The figure shows three views and two pictorial views of one solid part (mm, origin at its lowest corner). Answer the questions. A direction names the side the tool comes from. Coordinates: 2 decimals unless noted, no trailing zeros. Loops run counter-clockwise (first coordinate to the right, second up) from the corner with the lowest first, then second, coordinate; pieces in that order, holes last. Notation, with made-up numbers: M 12,-16 L 25,-16 A17 cw 25,5 Z; hole C 22.5,59 d5. An arc over 180 degrees is marked long. Return JSON: item names as keys, results as strings. Group by question number.
1. The mould has two halves that part along X. Classify the marked faces 4, 5 and 6: pulls with the +X half, pulls with the -X half, needs draft (parallel to the pull), parting line crosses it, or undercut.
2. Given P1, Ø4.5, axis at x = 39, z = 47, coming from the +Y side; P2, Ø1, axis at y = 31, z = 44.5, coming from the -X side; P3, Ø6, axis at y = 10.5, z = 32.5, coming from the -X side, each flat-ended and moving along its own axis, determine where each tip first touches the part or whether it passes through.
3. Section C-C (z = 11.5) is taken. Write down the section's boundary in (x, y), then the cut area to 3 significant figures.
4. Section B-B (y = 45) is taken. Write down the section's boundary in (x, z), then the cut area to 3 significant figures.
5. Section D-D (x = 66) is taken. Write down the section's boundary in (y, z) (1 decimal).
6. Section A-A (z = 28.5) is taken. Write down the section's boundary in (x, y), then the cut area to 3 significant figures.
7. Straight lines are drawn through the part: L1, parallel to Z at x = 66, y = 66.5; L2, parallel to Y at x = 49.5, z = 46.5; L3, parallel to Y at x = 24, z = 32.5. For each, find the intervals that lie inside material, in ascending order. Write a range as from..to.
8. Which of the six approach directions +Z, -Z, +X, -X, +Y, -Y give full straight-line access (tool end or side, diameter ignored) to the marked faces 1, 2 and 3?
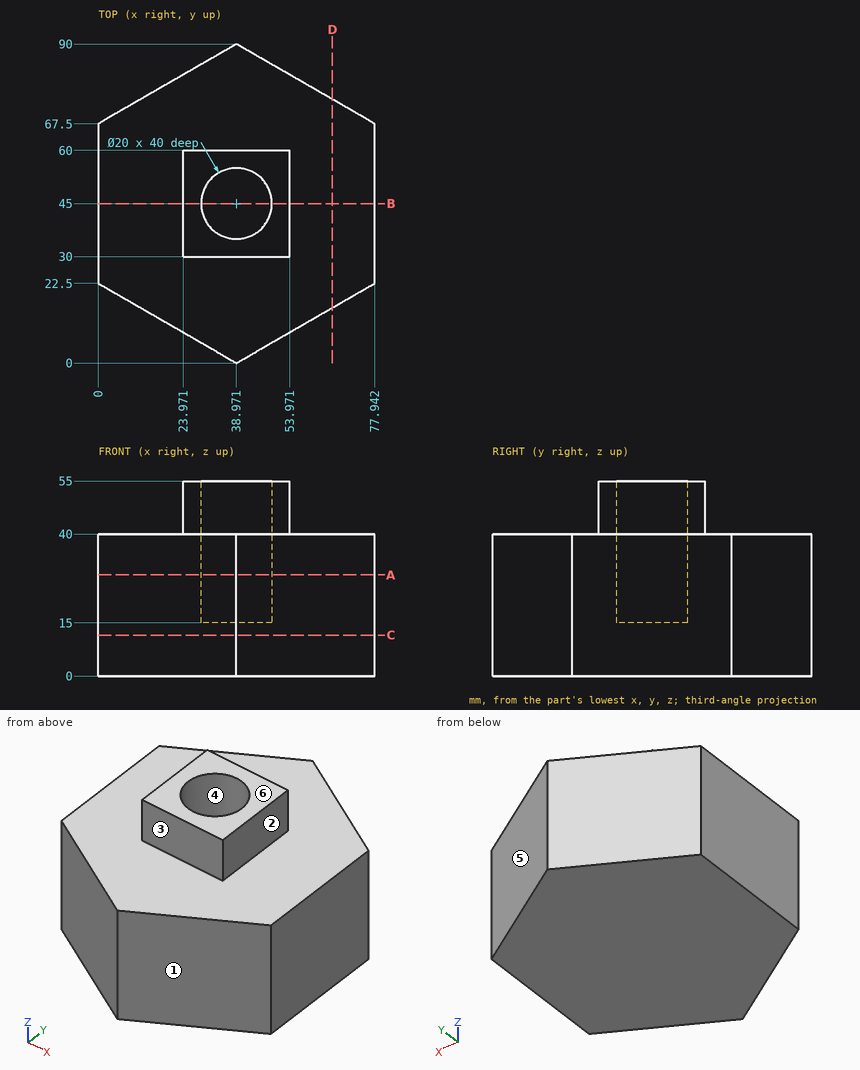
Worked out:
{
 "1": {"face 4": "undercut", "face 5": "pulls with the +X half", "face 6": "needs draft"},
 "2": {"P1": "y = 60", "P2": "x = 23.97", "P3": "x = 15.59"},
 "3": {"outline": "M 0,22.5 L 38.97,0 L 77.94,22.5 L 77.94,67.5 L 38.97,90 L 0,67.5 Z", "area": "5,260 mm^2"},
 "4": {"outline": "M 0,0 L 77.94,0 L 77.94,40 L 53.97,40 L 53.97,55 L 48.97,55 L 48.97,15 L 28.97,15 L 28.97,55 L 23.97,55 L 23.97,40 L 0,40 Z", "area": "2,770 mm^2"},
 "5": {"outline": "M 15.6,0 L 74.4,0 L 74.4,40 L 15.6,40 Z"},
 "6": {"outline": "M 0,22.5 L 38.97,0 L 77.94,22.5 L 77.94,67.5 L 38.97,90 L 0,67.5 Z; hole C 38.97,45 d20", "area": "4,950 mm^2"},
 "7": {"L1": "0..40", "L2": "30..60", "L3": "8.64..81.36"},
 "8": {"face 1": "+Z, -Z, +X, -Y", "face 2": "+Z, +X, +Y, -Y", "face 3": "+Z, +X, -X, -Y"}
}
